Verification items for the finished model (mm, model axes). A direction names the side the tool comes from. Round coordinates to 2 decimals unless told otherwise and drop trailing zeros. Write each loop counter-clockwise with the first axis right and the second up, starting at its lowest first coordinate (ties: lowest second). Pieces come first, ordered by that corner, then holes. Notation, with made-up numbers: (-25.5, 45) - (13.5, 45) arc R21 cw to (13.5, 74) - close; hole circle Ø8 at (-14, 28). An arc over 180 degrees is marked (long way). Answer as a JSON object with one key per item and string values. Group by question number.
1) Section check C-C (y = 3.7). Enter the section's corners in (x, z), then the cut area to 3 significant figures.
2) Section check B-B (z = -16). Enter the section's corners in (x, y), then the cut area to 3 significant figures.
3) Thickness scan on line 1 (X direction, y = 3.8, z = -20); line 2 (Z direction, x = -4.5, y = 3.35). Record the ranges inside material, lowest first.
4) Set-up check for faces 1 (the cylindrical face through (-89.43, 2.46, -89.4)), 2 (the flat face through (-43, 0, -92)): record each of +Z, -Z, +X, -X, +Y, -Y from which the full face is reachable in a straight line by a thin tool's end or side.
5) Section check A-A (x = -41). Enter the section's corners in (y, z).
6) Mould release check, pull along Z, two halves, no side actions. Record for faces 3 (the flat face through (0, 2, -48)), 4 (the cylindrical face through (-1, 3, -92)), 5 (the flat face through (-46, 3, -90)): +Z half, -Z half, draft (parallel to the pull), parting line (faces both ways), or undercut.
Autodesk Inventor part; units mm, degrees
ref_plane "YZ Plane" through (0, 0, 0) normal (1, 0, 0) x (0, 1, 0)
ref_plane "XZ Plane" through (0, 0, 0) normal (0, 1, 0) x (-1, 0, 0)
ref_plane "XY Plane" through (0, 0, 0) normal (0, 0, 1) x (1, 0, 0)
sketch "Sketch1" plane through (0, 0, 0) normal (0, 1, 0) x (-1, 0, 0)
  line L0 (0, 0) -> (94, 0)
  line L1 (94, 0) -> (94, -94)
  line L2 (94, -94) -> (0, -94)
  line L3 (0, -94) -> (0, 0)
  dimension "d0" = 94
  dimension "d1" = 94
extrude "Extrusion1" add sketch "Sketch1" along normal blind 5
sketch "Sketch2" plane through (0, 5, 0) normal (0, 1, 0) x (1, 0, 0)
  line L0 (-90, 4) -> (-4, 4)
  line L1 (-4, 4) -> (-4, 90)
  line L2 (-4, 90) -> (-90, 90)
  line L3 (-90, 90) -> (-90, 4)
  line L4 (0, 94) -> (-94, 94)
  line L5 (-94, 94) -> (-94, 0)
  line L6 (-94, 0) -> (0, 0)
  line L7 (0, 0) -> (0, 94)
  dimension "d4" = 4
  dimension "d5" = 4
  dimension "d6" = 4
  dimension "d7" = 4
extrude "Extrusion2" cut sketch "Sketch2" against normal blind 5 contours L3 L2 L1 L0
fillet "Fillet1" radius 5 4 edges at (-94, 2.5, -94) (0, 2.5, 0) (0, 2.5, -94) (-94, 2.5, 0)
sketch "Sketch3" plane through (0, 5, 0) normal (0, 1, 0) x (1, 0, 0)
  line L0 (-91.5, 91.5) -> (-2.5, 91.5) construction
  line L1 (-2.5, 91.5) -> (-2.5, 2.5) construction
  line L2 (-2.5, 2.5) -> (-91.5, 2.5) construction
  line L3 (-91.5, 2.5) -> (-91.5, 91.5) construction
  line L4 (0, 5) -> (0, 89)
  line L5 (-5, 94) -> (-89, 94)
  line L6 (-94, 89) -> (-94, 5)
  line L7 (-89, 0) -> (-5, 0)
  point P0 (0, 0)
  dimension "d11" = 2.5
  dimension "d12" = 2.5
  dimension "d13" = 2.5
  dimension "d14" = 2.5
fillet "Fillet2" radius 2 4 edges at (-90, 2.5, -90) (-4, 2.5, -90) (-4, 2.5, -4) (-90, 2.5, -4)
properties part number "Adult fly trap middle"
Returned:
{
 "1": {"outline": "(-94, -89) arc R5 ccw to (-89, -94) - (-5, -94) arc R5 ccw to (0, -89) - (0, -5) arc R5 ccw to (-5, 0) - (-89, 0) arc R5 ccw to (-94, -5) - close; hole (-90, -88) arc R2 ccw to (-88, -90) - (-6, -90) arc R2 ccw to (-4, -88) - (-4, -6) arc R2 ccw to (-6, -4) - (-88, -4) arc R2 ccw to (-90, -6) - close", "area": "1,420 mm2"},
 "2": {"outline": "(-94, 0) - (-90, 0) - (-90, 5) - (-94, 5) - close; (-4, 0) - (0, 0) - (0, 5) - (-4, 5) - close", "area": "40.0 mm2"},
 "3": {"line 1": "-94 to -90, -4 to 0", "line 2": "-93.97 to -89.32, -4.68 to -0.03"},
 "4": {"face 1": "+Y, -Y", "face 2": "+Z, -Z, +X, -X, -Y"},
 "5": {"outline": "(0, -94) - (5, -94) - (5, -90) - (0, -90) - close; (0, -4) - (5, -4) - (5, 0) - (0, 0) - close"},
 "6": {"face 3": "draft", "face 4": "-Z half", "face 5": "undercut"}
}
